```python
from build123d import *

# Parameters (mm, degrees)
BOSS_EXTRUDE1_DEPTH = 76.2
BOSS_EXTRUDE2_DEPTH = 5


with BuildPart() as part:
    # Sketch1 → Boss-Extrude1 (new body)
    with BuildSketch(Plane(origin=(0, 0, 0), x_dir=(1, 0, 0), z_dir=(0, 1, 0))):
        with BuildLine():
            ThreePointArc((12.330666952, 36.049475066), (0, 25.6), (-12.330666952, 36.049475066))
            ThreePointArc((-12.330666953, 36.049475066), (0, -38.1), (12.330666953, 36.049475066))
        make_face()
        with BuildLine():
            ThreePointArc((15.189386988, 29.409055118), (0, -33.1), (-15.189386988, 29.409055118))
            ThreePointArc((-15.189386988, 29.409055118), (0, 20.6), (15.189386988, 29.409055118))
        make_face(mode=Mode.SUBTRACT)
    extrude(amount=BOSS_EXTRUDE1_DEPTH)

    # Sketch1<3> → Boss-Extrude2 (add)
    with BuildSketch(Plane(origin=(0, 0, 0), x_dir=(1, 0, 0), z_dir=(0, 1, 0))):
        with BuildLine():
            ThreePointArc((33.1, 0), (28.269937295, 17.216870951), (15.189386988, 29.409055118))
            ThreePointArc((15.189386988, 29.409055118), (0, 20.6), (-15.189386988, 29.409055118))
            ThreePointArc((-15.189386988, 29.409055118), (-17.216870951, -28.269937295), (33.1, 0))
        make_face()
    extrude(amount=BOSS_EXTRUDE2_DEPTH)


solid = part.part
```
The model under review builds one solid part; all positions refer to its coordinate system, in mm. A direction names the side the tool comes from. Give positions to 0.01 mm unless a question says otherwise; leave off trailing zeros. Write each loop counter-clockwise with the first axis right and the second up, starting at its lowest first coordinate (ties: lowest second). Pieces come first, ordered by that corner, then holes. Notation, with made-up numbers: (59, 24.25) - (69, 24.25) arc R18 cw to (69, 52.25) - close; hole circle Ø2 at (63, 74). An arc over 180 degrees is marked (long way). Answer in a Markdown table with one row per item. Add a question column.
1. We need section C-C on y = 28. Write out the cut boundary in (x, z).
2. We need section B-B on x = -8. Write out the cut boundary in (y, z).
3. We need section D-D on z = -22. Write out the cut boundary in (x, y), then the cut area to 3 significant figures.
4. Insertion check: P1, Ø5, axis at y = 68.5, z = 17, coming from the +X side; P2, Ø4, axis at x = -4.5, y = 27.5, coming from the +Z side; P3, Ø2, axis at x = 28, y = 32.5, coming from the +Z side; P4, Ø10, axis at x = -9.5, y = 22.5, coming from the -Z side. Each pin has a flat end and moves straight along its axis. Give the tip position at first contact, or say it passes through.
5. Draft analysis for pull direction Z (two halves, no side actions). For faces 1 (the cylindrical face through (-0.26, 40.1, -20.6)), 2 (the flat face through (-3, 76.2, -21.1)), 3 (the cylindrical face through (1.235, 40.102, 33.077)), 4 (the cylindrical face through (-1.5, 37.57, 38.07)), state which applies: +Z half, -Z half, draft (parallel to the pull), parting line (faces both ways), or undercut.
6. We need section A-A on z = 0. Write out the cut boundary in (x, y).
7. Wall thickness on line 1 along X through (y, z) = (38.5, 0); line 2 along X through (y, z) = (23, 13); line 3 along X through (y, z) = (47.5, -27.5): over which ranges is each line inside the solid? List them lowest first. Write a range as [from, to].
8. Tool access review of faces 5 (the flat face through (0, 5, 1)), 6 (the flat face through (-1, 0, 1)): name each direction out of +Z, -Z, +X, -X, +Y, -Y from which nothing blocks a thin tool from reaching the whole face with its end or side.
Ans:
| question | item | result |
|---|---|---|
| 1 | outline | (-12.33, -36.05) arc R12.5 cw to (12.33, -36.05) arc R38.1 ccw (long way) to start; hole (-15.19, -29.41) arc R17.5 cw to (15.19, -29.41) arc R33.1 ccw (long way) to start |
| 2 | outline | (0, -28.5) - (76.2, -28.5) - (76.2, -22.54) - (5, -22.54) - (5, 32.12) - (76.2, 32.12) - (76.2, 37.25) - (0, 37.25) - close |
| 3 | outline | (-31.11, 0) - (31.11, 0) - (31.11, 76.2) - (24.73, 76.2) - (24.73, 5) - (6.86, 5) - (6.86, 76.2) - (-6.86, 76.2) - (-6.86, 5) - (-24.73, 5) - (-24.73, 76.2) - (-31.11, 76.2) - close |
| 3 | area | 2,200 mm^2 |
| 4 | P1 | stops at x = 35.23 |
| 4 | P2 | stops at z = 38.02 |
| 4 | P3 | stops at z = 26.88 |
| 4 | P4 | stops at z = -36.05 |
| 5 | face 1 | undercut |
| 5 | face 2 | draft |
| 5 | face 3 | undercut |
| 5 | face 4 | parting line |
| 6 | outline | (-38.1, 0) - (38.1, 0) - (38.1, 76.2) - (33.1, 76.2) - (33.1, 5) - (-33.1, 5) - (-33.1, 76.2) - (-38.1, 76.2) - close |
| 7 | line 1 | x = [-38.1, -33.1], [33.1, 38.1] |
| 7 | line 2 | x = [-35.81, -30.44], [30.44, 35.81] |
| 7 | line 3 | x = [-26.37, -18.42], [-13.92, -6.62], [6.62, 13.92], [18.42, 26.37] |
| 8 | face 5 | +Y |
| 8 | face 6 | +Z, -Z, +X, -X, -Y |
